Geometry: final body of the model. Coordinates: model frame, mm. Round coordinates to 2 decimals unless told otherwise and drop trailing zeros. Order: outer loops, then holes, each group sorted by start corner. A loop starts at its lowest first (then second) coordinate and runs counter-clockwise, first axis right, second up. Notation, with made-up numbers: (62, -31.75) - (98, -31.75) arc R9 cw to (98, -23.75) - close; hole circle Ø2 at (-18.5, 85). An arc over 180 degrees is marked (long way). Put each result on its own line as item: value. Start each with the question number.
(1) Section C-C (z = 8.75). Output: boundary loops of the cut face in (x, y) (3 decimals), and give its area (3 significant figures).
(2) Pin query (flat end, axial travel): P1, Ø4, axis at x = -2.5, z = 10, coming from the +Y side; P2, Ø8, axis at y = -5, z = 4.5, coming from the +X side; P3, Ø1.5, axis at x = -1.5, z = -1, coming from the +Y side. Return the tip coordinate at first contact, or that it passes through.
(3) Section B-B (y = -15.25). Output: boundary loops of the cut face in (x, z) (3 decimals).
(4) Pull-direction query (Z, two-part tool) for faces 1 (the face through (-3.948, -3.027, 6.93)), 2 (the face through (-4.345, -3.331, 0.986)); classes: released by +Z, released by -Z, zero draft, split by the parting line, or undercut.
(5) Section D-D (y = -1). Count the separate pieces of the cut face and the enclosed holes in it, and give its area (3 significant figures).
(6) Section A-A (x = 0). Output: boundary loops of the cut face in (y, z) (3 decimals), and give its area (3 significant figures).
(7) Material intervals for L1, parallel to X at y = -0.25, z = -1.25; L2, parallel to Z at x = 2.5, y = -4.5; L3, parallel to Z at x = -2, y = -3.75, sorted ascending. Write a range as [from, to].
from build123d import *

# Parameters (mm, degrees)
F0_R     = 5.475
F1_DEPTH = 2
F2_R     = 4.975
F3_DEPTH = 10
F6_R     = 0.25


with BuildPart() as f1:
    # F0 (on Top) → F1 (new body)
    with BuildSketch(Plane.XY):
        Circle(F0_R)
    extrude(amount=F1_DEPTH)

    # F2 (on face) → F3 (join)
    with BuildSketch(Plane.XY.offset(2)):
        Circle(F2_R)
    extrude(amount=F3_DEPTH)

    # F4 (on Front) → F5 (revolve)
    with BuildSketch(Plane.XZ):
        with BuildLine():
            Line((0, 17), (0, 12))
            Line((0, 12), (5, 12))
            ThreePointArc((5, 12), (3.5355339059, 15.5355339059), (0, 17))
        make_face()
    revolve(axis=Axis((0, 0, 14.5), (0, 0, 1)))

    # F9: sweep along a path in F8
    with BuildLine(Plane.YZ.offset(1.974)) as f9_path:
        Line((-23, -4), (-4, -4))
        ThreePointArc((-4, -4), (-1.1715728753, -2.8284271247), (0, 0))
    # F6 (on Top) → F9 (sweep)
    with BuildSketch(Plane.XY):
        with Locations((-1.975, 0)):
            Circle(F6_R)
        with Locations((1.975, 0)):
            Circle(F6_R)
        with Locations((-0.659, 0)):
            Circle(F6_R)
        with Locations((0.659, 0)):
            Circle(F6_R)
    sweep(path=f9_path.line)


solid = f1.part
Checks:
1. outline: circle Ø9.95 at (0, 0)
1. area: 77.8 mm²
2. P1: stops at y = 4.95
2. P2: stops at x = 5.14
2. P3: stops at y = 0.23
3. outline: circle Ø0.5 at (-1.975, -4); circle Ø0.5 at (-0.659, -4); circle Ø0.5 at (0.659, -4); circle Ø0.5 at (1.975, -4)
4. face 1: undercut
4. face 2: zero draft
5. separate pieces: 5
5. enclosed holes: 0
5. area: 158 mm²
6. outline: (-5.475, 0) - (5.475, 0) - (5.475, 2) - (4.975, 2) - (4.975, 12) - (5, 12) arc R5 ccw to (-5, 12) - (-4.975, 12) - (-4.975, 2) - (-5.475, 2) - close
6. area: 161 mm²
7. L1: x = [-2.22, -1.73], [-0.9, -0.41], [0.41, 0.9], [1.73, 2.22]
7. L2: z = [0, 2]
7. L3: z = [-4.24, -3.74], [0, 14.63]
